Check sheet for the modelled part. Datum: model origin and axes. Units: mm. A direction names the side the tool comes from. Round coordinates to 2 decimals unless told otherwise and drop trailing zeros. Write each loop counter-clockwise with the first axis right and the second up, starting at its lowest first coordinate (ties: lowest second). Pieces come first, ordered by that corner, then holes.
Item 1: Cross-section at A-A on x = 0. Enter the section's corners in (y, z).
Item 2: Material ranges on line 1 (Y direction, x = -3, z = -12); line 2 (Y direction, x = 4, z = 2); line 3 (Z direction, x = -6, y = 9), recorded low to high.
Item 3: Go/stop test with flat-tipped pins: pin 1 Ø12 at (y, z) = (21.5, 7.5) entering from -X; pin 2 Ø12 at (x, z) = (10.5, -4.5) entering from +Y; pin 3 Ø5 at (y, z) = (13.5, 3) entering from -X. Record where each tip stops, or that it passes through.
Item 4: Cross-section at C-C on y = 37. Enter the section's corners in (x, z).
Item 5: Tool access check on faces 1 (the flat face through (0, 67.5, 0)), 2 (the cylindrical face through (-0.34, 61.16, 1.55)). Record the directions out of +Z, -Z, +X, -X, +Y, -Y that give a thin tool (end or side, any length) a straight path to the whole face; none if there is none.
Item 6: Cross-section at B-B on z = 0. Enter the section's corners in (x, y), plus the area to 3 significant figures.
Item 7: Cross-section at D-D on x = -5. Enter the section's corners in (y, z).
from build123d import *

# Parameters (mm, degrees)
SKETCH1_R           = 18
BOSS_EXTRUDE1_DEPTH = 50
BOSS_EXTRUDE2_START = 50
SKETCH2_R           = 6.5
BOSS_EXTRUDE2_DEPTH = 5
BOSS_EXTRUDE3_START = 55
SKETCH3_R           = 1.5875
BOSS_EXTRUDE3_DEPTH = 12.5


with BuildPart() as part:
    # Sketch1 → Boss-Extrude1 (new body)
    with BuildSketch(Plane(origin=(0, 0, 0), x_dir=(1, 0, 0), z_dir=(0, 1, 0))):
        Circle(SKETCH1_R)
    extrude(amount=BOSS_EXTRUDE1_DEPTH)

    # Sketch2 → Boss-Extrude2 (add)
    with BuildSketch(Plane(origin=(0, 0, 0), x_dir=(1, 0, 0), z_dir=(0, 1, 0)).offset(BOSS_EXTRUDE2_START)):
        Circle(SKETCH2_R)
    extrude(amount=BOSS_EXTRUDE2_DEPTH)

    # Sketch3 → Boss-Extrude3 (add)
    with BuildSketch(Plane(origin=(0, 0, 0), x_dir=(1, 0, 0), z_dir=(0, 1, 0)).offset(BOSS_EXTRUDE3_START)):
        Circle(SKETCH3_R)
    extrude(amount=BOSS_EXTRUDE3_DEPTH)


solid = part.part
Response values:
1. outline: (0, -18) - (50, -18) - (50, -6.5) - (55, -6.5) - (55, -1.59) - (67.5, -1.59) - (67.5, 1.59) - (55, 1.59) - (55, 6.5) - (50, 6.5) - (50, 18) - (0, 18) - close
2. line 1: y = 0 to 50
2. line 2: y = 0 to 55
2. line 3: z = -16.97 to 16.97
3. pin 1: stops at x = -17.94
3. pin 2: stops at y = 55
3. pin 3: stops at x = -17.99
4. outline: circle Ø36 at (0, 0)
5. face 1: +Z, -Z, +X, -X, +Y
5. face 2: +Y
6. outline: (-18, 0) - (18, 0) - (18, 50) - (6.5, 50) - (6.5, 55) - (1.59, 55) - (1.59, 67.5) - (-1.59, 67.5) - (-1.59, 55) - (-6.5, 55) - (-6.5, 50) - (-18, 50) - close
6. area: 1,900 mm2
7. outline: (0, -17.29) - (50, -17.29) - (50, -4.15) - (55, -4.15) - (55, 4.15) - (50, 4.15) - (50, 17.29) - (0, 17.29) - close
